Check sheet for the modelled part. Datum: model origin and axes. Units: mm. Face numbers are marked on the shaded views. A direction names the side the tool comes from. Round coordinates to 2 decimals unless told otherwise and drop trailing zeros. Order: outer loops, then holes, each group sorted by start corner. A loop starts at its lowest first (then second) coordinate and runs counter-clockwise, first axis right, second up. Notation, with made-up numbers: M 37,36.25 L 63,36.25 A6 ccw 63,47.25 Z; hole C 75.5,-26.5 d6. An arc over 180 degrees is marked long. One line per item, written item: value. Start each with the question number.
(1) Cross-section at B-B, the plane x = 15. Enter the section's corners in (y, z), and give its area (3 significant figures).
(2) Cross-section at A-A, the plane z = 38. Enter the section's corners in (x, y), and give its area (3 significant figures).
(3) Access from +Z, -Z, +X, -X, +Y, -Y to the whole of each face (thin tool, end or side, straight path). Record for the marked faces 5, 6, 7 and 8.
(4) Thickness scan on L1, parallel to X at y = 4, z = 14; L2, parallel to X at y = 10.5, z = 14.5; L3, parallel to X at y = 31, z = 21.5. Record the ranges inside material, lowest first.
(5) Depth check by flat-ended pin: pin 1 Ø1.8 at (y, z) = (3, 24.5) entering from +X; pin 2 Ø0.8 at (x, y) = (35.5, 46.5) entering from -Z; pin 3 Ø2.5 at (x, y) = (-24.5, 3) entering from +Z. Enter the tip coordinate at first touch or a pass-through.
(6) Cross-section at C-C, the plane y = 10. Enter the section's corners in (x, z), and give its area (3 significant figures).
(7) Release check for a two-part mould opening along X. For the marked faces 1, 2, 3 and 4 record: released by +X, released by -X, zero draft, split by the parting line, or undercut.
(8) Cross-section at D-D, the plane x = -25. Enter the section's corners in (y, z).
from build123d import *

# Parameters (mm, degrees)
BOSS_EXTRU_1_DEPTH           = 39
ESQUISSE2_W                  = 36
ESQUISSE2_H                  = 35
ENL_V_MAT_EXTRU_1_DEPTH      = 69.490875305
ENL_V_MAT_EXTRU_2_DEPTH      = 7.5
ENL_V_MAT_EXTRU_2_DEPTH_BACK = 39
ESQUISSE3_W                  = 3
ESQUISSE3_H                  = 32
ESQUISSE5_W                  = 7.5
ESQUISSE5_H                  = 28.5
ENL_V_MAT_EXTRU_3_DEPTH      = 66.024995194
ESQUISSE6_W                  = 2
ESQUISSE6_H                  = 2
CONG_2_R                     = 1
BOSS_EXTRU_3_DEPTH           = 7.5
CHANFREIN1_SIZE              = 5
CHANFREIN1_SIZE_2            = 7.699324819
ESQUISSE9_W                  = 5
ESQUISSE9_H                  = 28.629443051
ENL_V_MAT_EXTRU_4_DEPTH      = 6
ESQUISSE10_W                 = 16
ESQUISSE10_H                 = 28.629443051
ENL_V_MAT_EXTRU_6_DEPTH      = 76.996780236


# Some blends are built 0.0001 mm under size
with BuildPart() as part:
    # Esquisse1 → Boss.-Extru.1 (new body)
    with BuildSketch(Plane.XY):
        Polygon((-38.5, 0), (0, 0), (0, 12), (-31, 12), (-31, 47), (-38.5, 47), align=None)
    extrude(amount=BOSS_EXTRU_1_DEPTH)

    # Esquisse2 → Enlèv. mat.-Extru.1 (cut, through all)
    with BuildSketch(Plane(origin=(-31, 0, 0), x_dir=(0, 0, -1), z_dir=(1, 0, 0))):
        with Locations((-18, 29.5)):
            Rectangle(ESQUISSE2_W, ESQUISSE2_H)
    extrude(amount=-ENL_V_MAT_EXTRU_1_DEPTH, mode=Mode.SUBTRACT)

    # Esquisse3 → Enlèv. mat.-Extru.2 (cut, two sides: drawn at the far end of the back side and taken through both)
    with BuildSketch(Plane(origin=(0, 0, 36), x_dir=(-1, 0, 0), z_dir=(0, 0, -1)).offset(-ENL_V_MAT_EXTRU_2_DEPTH_BACK)):
        with Locations((33.5, 28)):
            Rectangle(ESQUISSE3_W, ESQUISSE3_H)
    extrude(amount=ENL_V_MAT_EXTRU_2_DEPTH + ENL_V_MAT_EXTRU_2_DEPTH_BACK, mode=Mode.SUBTRACT)

    # Esquisse5 → Enlèv. mat.-Extru.3 (cut, through all)
    with BuildSketch(Plane(origin=(0, 12, 0), x_dir=(1, 0, 0), z_dir=(0, 1, 0))):
        with Locations((-34.75, -21.75)):
            Rectangle(ESQUISSE5_W, ESQUISSE5_H)
    extrude(amount=-ENL_V_MAT_EXTRU_3_DEPTH, mode=Mode.SUBTRACT)

    # Balayage3: sweep along a path in Esquisse7
    with BuildLine(Plane(origin=(0, 47, 0), x_dir=(1, 0, 0), z_dir=(0, 1, 0))) as balayage3_path:
        Line((-37.5, -39), (-37.5, -41.903703094))
        ThreePointArc((-37.5, -41.903703094), (-34.75, -44.653703094), (-32, -41.903703094))
        Line((-32, -41.903703094), (-32, -39))
    # Esquisse6 → Balayage3 (sweep)
    with BuildSketch(Plane.XY.offset(39)):
        with Locations((-37.5, 46)):
            Rectangle(ESQUISSE6_W, ESQUISSE6_H)
    sweep(path=balayage3_path.line)

    # Congé2
    cong_2_edges = [part.edges().sort_by_distance(p)[0] for p in [
        (-31, 47, 38.951851547),
        (-38.5, 47, 38.951851547),
        (-31, 45, 40.451851547),
        (-33, 47, 40.451851547),
        (-38.5, 45, 40.451851547),
        (-36.5, 47, 40.451851547),
        (-33, 45, 40.451851547),
        (-34.75, 47, 45.653703094),
        (-34.75, 45, 45.653703094),
        (-34.75, 45, 43.653703094),
        (-34.75, 47, 43.653703094),
        (-36.5, 45, 40.451851547),
    ]]
    fillet(cong_2_edges, radius=CONG_2_R - 0.0001)  # a hair under: the kernel refuses the full size

    # Esquisse8 → Boss.-Extru.3 (add)
    with BuildSketch(Plane.ZY.offset(38.5)):
        Polygon((36, 46), (0, 12), (2, 12), (36, 44), align=None)
    extrude(amount=-BOSS_EXTRU_3_DEPTH)

    # Chanfrein1
    # the kernel refuses this chamfer: 7.699324819, 5 mm, written as the material it takes off along each edge
    with BuildSketch(Plane(origin=(-38.5, 31.898450737, 7.5), x_dir=(-0.04991856572298867, 0, -0.9987532912567346), z_dir=(0, -1, 0))) as chanfrein1_piece_1_section:
        Polygon((CHANFREIN1_SIZE * 0.998753291257, CHANFREIN1_SIZE * 0.049918565723), (-CHANFREIN1_SIZE_2 * 0.0499185657235, CHANFREIN1_SIZE_2 * 0.998753291266), (0, 0), align=None)
    chanfrein1_piece_1 = extrude(amount=51.796901474, mode=Mode.PRIVATE)
    chanfrein1_piece_1 = split(chanfrein1_piece_1, bisect_by=Plane(origin=(-31, 6, 5.832244488), z_dir=(-1, 0, 0)), keep=Keep.TOP, mode=Mode.PRIVATE)
    chanfrein1_piece_1 = split(chanfrein1_piece_1, bisect_by=Plane(origin=(-35.936911742, 11.0942578, 1.037648912), z_dir=(0, -0.7281999926928029, 0.685364699004991)), keep=Keep.TOP, mode=Mode.PRIVATE)
    add(chanfrein1_piece_1, mode=Mode.SUBTRACT)

    # Esquisse9 → Enlèv. mat.-Extru.4 (cut)
    with BuildSketch(Plane.XZ):
        with Locations((-23.5, 21.685278474)):
            Rectangle(ESQUISSE9_W, ESQUISSE9_H)
    extrude(amount=-ENL_V_MAT_EXTRU_4_DEPTH, mode=Mode.SUBTRACT)

    # Esquisse10 → Enlèv. mat.-Extru.6 (cut, through all)
    with BuildSketch(Plane.XZ):
        with Locations((-8, 21.685278474)):
            Rectangle(ESQUISSE10_W, ESQUISSE10_H)
    extrude(amount=-ENL_V_MAT_EXTRU_6_DEPTH, mode=Mode.SUBTRACT)

    # Symétrie1: part across plane


with BuildPart() as part_1:
    add(part.part)
    add(part.part.mirror(Plane(origin=(0, 12, 39), x_dir=(0, 0, 1), z_dir=(1, 0, 0))))


solid = part_1.part
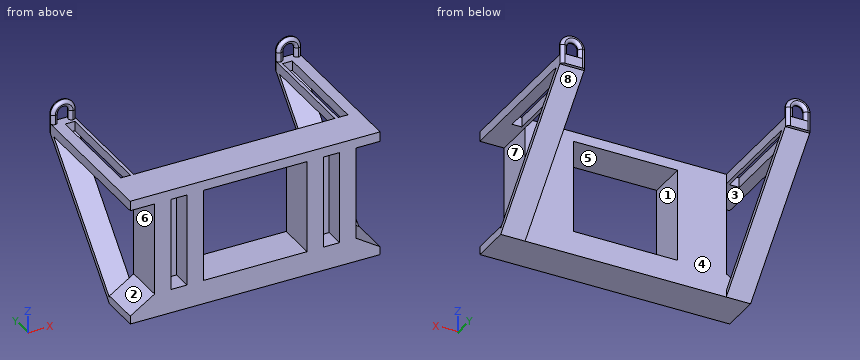
Values found:
1. outline: M 0,0 L 12,0 L 12,7.37 L 0,7.37 Z; M 0,36 L 12,36 L 12,39 L 0,39 Z
1. area: 124 mm^2
2. outline: M -38.5,0 L 38.5,0 L 38.5,46 A1 ccw 37.5,47 L 32,47 A1 ccw 31,46 L 31,12 L -31,12 L -31,46 A1 ccw -32,47 L -37.5,47 A1 ccw -38.5,46 Z; hole M -35,12 L -32,12 L -32,44 L -35,44 Z; hole M 32,12 L 35,12 L 35,44 L 32,44 Z
2. area: 1,260 mm^2
3. face 5: +Y, -Y
3. face 6: -X, -Y
3. face 7: +X, -Y
3. face 8: -Z, +X, -X, +Y
4. L1: -31 to -26, -21 to -16, 16 to 21, 26 to 31
4. L2: -31 to -16, 16 to 31
4. L3: -38.5 to -31, 31 to 38.5
5. pin 1: x = 31
5. pin 2: z = 36
5. pin 3: z = 39
6. outline: M -38.5,0 L 38.5,0 L 38.5,2.5 L 31,7.37 L 31,36 L 38.5,36 L 38.5,39 L -38.5,39 L -38.5,36 L -31,36 L -31,7.37 L -38.5,2.5 Z; hole M -16,7.37 L 16,7.37 L 16,36 L -16,36 Z
6. area: 1,620 mm^2
7. face 1: undercut
7. face 2: released by -X
7. face 3: zero draft
7. face 4: undercut
8. outline: M 0,0 L 12,0 L 12,39 L 0,39 L 0,36 L 6,36 L 6,7.37 L 0,7.37 Z
